from build123d import *

# Parameters (mm, degrees)
CORTE_EXTRUS_O1_DEPTH      = 4
CHANFRO1_SIZE              = 1
CORTE_EXTRUS_O2_DEPTH      = 78.951908251
CORTE_EXTRUS_O2_DEPTH_BACK = 12
ESBO_O3_R                  = 1.5
CORTE_EXTRUS_O3_START      = -12
ESBO_O3_5_R                = 1.5
CORTE_EXTRUS_O3_DEPTH      = 66.951908251
CHANFRO2_SIZE              = 2
ESBO_O4_R                  = 1.25
CORTE_EXTRUS_O4_DEPTH      = 6
CORTE_EXTRUS_O5_REACH      = 79.952
ESBO_O4_3_R                = 4


with BuildPart() as part:
    # Esboço1 → Revolução1 (revolve)
    with BuildSketch(Plane.XY, mode=Mode.PRIVATE) as revolu_o1_sk:
        Polygon((44.5, 0), (44.5, 8), (36.3, 8), (36.3, 18.5), (33.7, 18.5), (33.7, 22), (36.3, 22), (36.3, 27), (33.7, 27), (33.7, 30.5), (36.3, 30.5), (36.3, 35.5), (33.7, 35.5), (33.7, 39), (36.3, 39), (36.3, 46), (22, 46), (22, 12), (0, 12), (0, 0), align=None)
    revolve(revolu_o1_sk.sketch.rotate(Axis((0, 0, 0), (0, 1, 0)), 90), axis=Axis((0, 0, 0), (0, 1, 0)))

    # Esboço2 → Corte-extrusão1 (cut)
    with BuildSketch(Plane(origin=(0, 8, 0), x_dir=(1, 0, 0), z_dir=(0, 1, 0))):
        with BuildLine():
            Line((5, 45.5), (5, 43.5))
            ThreePointArc((5, 43.5), (0, 38.5), (-5, 43.5))
            Line((-5, 43.5), (-5, 45.5))
            ThreePointArc((-5, 45.5), (0, 50.5), (5, 45.5))
        make_face()
        with BuildLine():
            Line((5, -45.5), (5, -43.5))
            ThreePointArc((5, -43.5), (0, -38.5), (-5, -43.5))
            Line((-5, -43.5), (-5, -45.5))
            ThreePointArc((-5, -45.5), (0, -50.5), (5, -45.5))
        make_face()
    extrude(amount=-CORTE_EXTRUS_O1_DEPTH, mode=Mode.SUBTRACT)

    # Chanfro1
    chanfro1_edges = [part.edges().sort_by_distance(p)[0] for p in [
        (0, 46, 36.3),
    ]]
    chamfer(chanfro1_edges, length=CHANFRO1_SIZE)

    # Esboço3 → Corte-extrusão2 (cut, two sides: drawn at the far end of the back side and taken through both)
    with BuildSketch(Plane.XZ.offset(-CORTE_EXTRUS_O2_DEPTH_BACK)):
        with Locations(Location((-27, 0, 0), (0, 0, 270))):
            Circle(ESBO_O3_R)
        with Locations(Location((27, 0, 0), (0, 0, 270))):
            Circle(ESBO_O3_R)
    extrude(amount=CORTE_EXTRUS_O2_DEPTH + CORTE_EXTRUS_O2_DEPTH_BACK, mode=Mode.SUBTRACT)

    # Esboço3<5> → Corte-extrusão3 (cut, through all)
    # profile 1 of 2: a face of its own
    with BuildSketch(Plane.XZ.offset(CORTE_EXTRUS_O3_START)):
        with BuildLine():
            Line((-27, 3.25), (-21.5, 3.25))
            ThreePointArc((-21.5, 3.25), (-18.25, 0), (-21.5, -3.25))
            Line((-21.5, -3.25), (-27, -3.25))
            ThreePointArc((-27, -3.25), (-30.25, 0), (-27, 3.25))
        make_face()
        with Locations(Location((-27, 0, 0), (0, 0, 270))):
            Circle(ESBO_O3_5_R, mode=Mode.SUBTRACT)
    # profile 2 of 2: a face of its own
    with BuildSketch(Plane.XZ.offset(CORTE_EXTRUS_O3_START)):
        with BuildLine():
            Line((27, 3.25), (21.5, 3.25))
            ThreePointArc((21.5, 3.25), (18.25, 0), (21.5, -3.25))
            Line((21.5, -3.25), (27, -3.25))
            ThreePointArc((27, -3.25), (30.25, 0), (27, 3.25))
        make_face()
        with Locations(Location((27, 0, 0), (0, 0, 270))):
            Circle(ESBO_O3_5_R, mode=Mode.SUBTRACT)
    extrude(amount=-CORTE_EXTRUS_O3_DEPTH, mode=Mode.SUBTRACT)


with BuildPart() as corte_extrus_o3_kept_piece:
    # of the separate pieces the step leaves, the one the design keeps (corte_extrus_o3_pieces_kept)
    add(part.part.solids().sort_by_distance((0, 45, -36.3))[0])

    # Chanfro2
    chanfro2_edges = [corte_extrus_o3_kept_piece.edges().sort_by_distance(p)[0] for p in [
        (0, 0, 44.5),
    ]]
    chamfer(chanfro2_edges, length=CHANFRO2_SIZE)

    # Esboço4 → Corte-extrusão4 (cut)
    with BuildSketch(Plane.XZ):
        with Locations(Location((-8.5, 7, 0), (0, 0, 270))):
            Circle(ESBO_O4_R)
        with Locations(Location((8.5, 7, 0), (0, 0, 270))):
            Circle(ESBO_O4_R)
    extrude(amount=-CORTE_EXTRUS_O4_DEPTH, mode=Mode.SUBTRACT)

    # Esboço4<3> → Corte-extrusão5 (cut, up to next)
    with BuildSketch(Plane.XZ, mode=Mode.PRIVATE) as corte_extrus_o5_sk1:
        with Locations(Location((0, -13, 0), (0, 0, 270))):
            Circle(ESBO_O4_3_R)
    corte_extrus_o5_tool1 = extrude(corte_extrus_o5_sk1.sketch, amount=-CORTE_EXTRUS_O5_REACH, mode=Mode.PRIVATE) & corte_extrus_o3_kept_piece.part
    add(corte_extrus_o5_tool1.solids().sort_by_distance((0, 0, -13))[0], mode=Mode.SUBTRACT)


solid = corte_extrus_o3_kept_piece.part
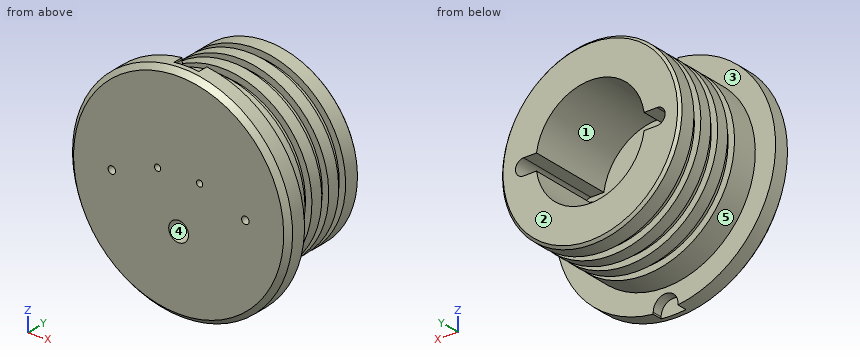
Geometry check sheet. Reference: the model listing, model coordinates, mm. Face numbers are marked on the shaded views. A direction names the side the tool comes from. Give positions to 0.01 mm unless a question says otherwise; leave off trailing zeros. Loops run counter-clockwise (first coordinate to the right, second up) from the corner with the lowest first, then second, coordinate; pieces in that order, holes last.
(1) Section check A-A on y = 24. Record the cut outline in (x, z), then the cut area to 3 significant figures.
From the geometry:
outline: circle Ø72.6 at (0, 0); hole (-27, -3.25) - (-21.76, -3.25) arc R22 ccw to (21.76, -3.25) - (27, -3.25) arc R3.25 ccw to (27, 3.25) - (21.76, 3.25) arc R22 ccw to (-21.76, 3.25) - (-27, 3.25) arc R3.25 ccw to start
area: 2,520 mm2
(2) Release check for a two-part mould opening along Z. For the marked faces 3, 4 and 5 record: released by +Z, released by -Z, zero draft, split by the parting line, or undercut.
From the geometry:
face 3: zero draft
face 4: undercut
face 5: split by the parting line
(3) Thickness scan on L1, parallel to X at y = 8.5, z = 0; L2, parallel to X at y = 6, z = 0; L3, parallel to Y at x = -32.5, z = 12.5. Record the ranges inside material, lowest first.
From the geometry:
L1: x = -36.3 to -28.5, -25.5 to 25.5, 28.5 to 36.3
L2: x = -44.5 to -28.5, -25.5 to 25.5, 28.5 to 44.5
L3: y = 0 to 18.5, 22 to 27, 30.5 to 35.5, 39 to 46
(4) Set-up check for the marked faces 1 and 2: record each of +Z, -Z, +X, -X, +Y, -Y from which the full face is reachable in a straight line by a thin tool's end or side.
From the geometry:
face 1: +Y
face 2: +Z, -Z, +X, -X, +Y
(5) Depth check by flat-ended pin: pin 1 Ø8 at (x, y) = (14, 39) entering from -Z; pin 2 Ø5 at (y, z) = (29.5, 17) entering from +X; pin 3 Ø2.5 at (x, z) = (27, 0) entering from -Y; pin 4 Ø2 at (x, y) = (-13.5, 23.5) entering from -Z. Enter the tip coordinate at first touch or a pass-through.
From the geometry:
pin 1: stops at z = -34.9
pin 2: stops at x = 33.19
pin 3: passes through
pin 4: stops at z = -34.08
(6) Section check B-B on z = 0. Count the separate pieces of the cut face and the enclosed holes in it, then the cut area to 3 significant figures.
From the geometry:
separate pieces: 3
enclosed holes: 0
area: 1,280 mm2
